Read the model definition and answer for the solid it produces. Units are mm, in the model's axes. Face numbers are marked on the shaded views. A direction names the side the tool comes from. Round coordinates to 2 decimals unless told otherwise and drop trailing zeros. Order: outer loops, then holes, each group sorted by start corner. A loop starts at its lowest first (then second) coordinate and runs counter-clockwise, first axis right, second up. Notation, with made-up numbers: M 25.5,-7 L 31.5,-7 A15 cw 31.5,14 Z; hole C 50.25,83.5 d5. An arc over 180 degrees is marked long. Answer as CSV lines item,"result".
```python
from build123d import *
from build123d.topology import SkipClean

# Parameters (mm, degrees)
SKETCH2_R           = 1.5
BOSS_EXTRUDE1_DEPTH = 3
SKETCH3_R           = 9.096048505
BOSS_EXTRUDE2_DEPTH = 1.2
FILLET1_R           = 1
CUT_EXTRUDE1_DEPTH  = 1.5
CUT_EXTRUDE2_START  = -1.5
CUT_EXTRUDE2_DEPTH  = 1.5
CUT_EXTRUDE3_DEPTH  = 5
MOVE_FACE1_BY       = 0.1
MOVE_FACE1_2_BY     = 0.1
MOVE_FACE1_3_BY     = 0.1


with BuildPart() as part:
    # Sketch2 → Boss-Extrude1 (new, symmetric)
    with BuildSketch(Plane(origin=(0, 0, 0), x_dir=(1, 0, 0), z_dir=(0, 1, 0))):
        with BuildLine():
            Line((-20.599560655, -3.593123858), (-21.028912901, -3.379903546))
            Line((-21.028912901, -3.379903546), (-21.254187526, 1.993220784))
            add(Edge.make_bspline(
                [(-21.254187526, 1.993220784), (-21.250081776, 2.377226096), (-21.195139063, 3.186038357), (-20.237966675, 3.678013728), (-19.626306607, 3.674971934), (-19.293061526, 3.554683236)],
                knots=[0.008573336, 0.008573336, 0.008573336, 0.008573336, 0.425411643, 0.645508579, 0.988655727, 0.988655727, 0.988655727, 0.988655727], degree=3))
            Line((-19.293061526, 3.554683236), (-19.293061526, -0.935875279))
            ThreePointArc((-19.293061526, -0.935875279), (-11.01478007, -15.867347151), (5.868677769, -18.402627716))
            ThreePointArc((5.868677769, -18.402627716), (8.914480471, -17.213611271), (11.689585214, -15.484603502))
            Line((11.689585214, -15.484603502), (16.248961374, -16.876941699))
            ThreePointArc((16.248961374, -16.876941699), (18.257558766, -15.774505508), (18.891422269, -13.572677609))
            Line((18.891422269, -13.572677609), (16.51986009, -9.867884272))
            ThreePointArc((16.51986009, -9.867884272), (18.681381592, -1.319406436), (16.449996012, 7.211101574))
            Line((16.449996012, 7.211101574), (17.928084104, 7.713187831))
            ThreePointArc((17.928084104, 7.713187831), (18.677006581, 8.400562387), (19.066466062, 9.339545863))
            Line((19.066466062, 9.339545863), (19.069212644, 11.701301235))
            ThreePointArc((19.069212644, 11.701301235), (18.53112158, 13.108816633), (17.413375201, 14.119402908))
            Line((17.413375201, 14.119402908), (16.248961374, 14.508827059))
            Line((16.248961374, 14.508827059), (17.314988377, 17.040275234))
            Line((17.314988377, 17.040275234), (-18.629227908, 17.040275234))
            Line((-18.629227908, 17.040275234), (-23.111573489, 16.669208858))
            ThreePointArc((-23.111573489, 16.669208858), (-24.534989581, 15.930034001), (-25.030823978, 14.404700893))
            Line((-25.030823978, 14.404700893), (-25.030823978, 12.70560175))
            ThreePointArc((-25.030823978, 12.70560175), (-24.756748057, 11.739888101), (-24.016241086, 11.062119787))
            Line((-24.016241086, 11.062119787), (-19.293061526, 9.00102042))
            Line((-19.293061526, 9.00102042), (-19.293061526, 5.839179653))
            Line((-19.293061526, 5.839179653), (-22.090684207, 5.839179653))
            ThreePointArc((-22.090684207, 5.839179653), (-22.935760928, 5.565442119), (-23.357392581, 4.783576625))
            Line((-23.357392581, 4.783576625), (-23.096619876, -3.253456456))
            Line((-23.096619876, -3.253456456), (-23.621531964, -3.576891157))
            ThreePointArc((-23.621531964, -3.576891157), (-23.831523214, -3.884927944), (-23.671952518, -4.221855504))
            Line((-23.671952518, -4.221855504), (-23.25143386, -4.644287186))
            Line((-23.25143386, -4.644287186), (-23.202937263, -6.523606801))
            add(Edge.make_bspline(
                [(-23.202937263, -6.523606801), (-23.190415125, -6.701394879), (-23.14585211, -7.158039831), (-22.604610265, -7.291644066), (-22.131088375, -7.301130698), (-21.611573501, -7.301182592), (-20.850084131, -7.060004854), (-20.915185829, -6.352757768), (-20.915665013, -6.081028816)],
                knots=[0, 0, 0, 0, 0.172348306, 0.293808545, 0.415161147, 0.571057182, 0.730620463, 1, 1, 1, 1], degree=3))
            Line((-20.915665013, -6.081028816), (-20.979073646, -4.568641575))
            Line((-20.979073646, -4.568641575), (-20.599560655, -4.155522335))
            ThreePointArc((-20.599560655, -4.155522335), (-20.467265038, -3.874323097), (-20.599560655, -3.593123858))
        make_face()
        with Locations(Location((16.153998691, -14.195749789, 0), (0, 0, 270))):
            Circle(SKETCH2_R, mode=Mode.SUBTRACT)
        with Locations(Location((-22.494848615, 13.810394624, 0), (0, 0, 270))):
            Circle(SKETCH2_R, mode=Mode.SUBTRACT)
        with Locations(Location((16.894563054, 10.777137226, 0), (0, 0, 270))):
            Circle(SKETCH2_R, mode=Mode.SUBTRACT)
    extrude(amount=BOSS_EXTRUDE1_DEPTH, both=True)

    # Sketch3 → Boss-Extrude2 (add)
    with BuildSketch(Plane(origin=(0, 3, 0), x_dir=(1, 0, 0), z_dir=(0, 1, 0))):
        with Locations(Location((3.73137128, -0.69899531, 0), (0, 0, 270))):
            Circle(SKETCH3_R)
    extrude(amount=BOSS_EXTRUDE2_DEPTH)

    # Fillet1
    fillet1_edges = [part.edges().sort_by_distance(p)[0] for p in [
        (3.73137128, 4.2, -8.397053195),
    ]]
    fillet(fillet1_edges, radius=FILLET1_R)

    # Sketch4 → Cut-Extrude1 (cut)
    with SkipClean():  # the faces are left unmerged after this step: merging them gives an invalid solid
        with BuildSketch(Plane(origin=(0, 3, 0), x_dir=(1, 0, 0), z_dir=(0, 1, 0))):
            Polygon((-19.293061526, 7.248655358), (-19.293061526, 22.083159944), (-29.904114882, 22.083159944), (-28.79317924, 8.663465276), align=None)
            with BuildLine():
                Line((17.65280475, 17.842473148), (14.40910217, 10.139793056))
                ThreePointArc((14.40910217, 10.139793056), (16.735981963, 6.675507155), (18.187015276, 2.762688645))
                Line((18.187015276, 2.762688645), (25.347732491, 2.045186791))
                Line((25.347732491, 2.045186791), (30.175625625, 15.043360613))
                Line((30.175625625, 15.043360613), (17.65280475, 17.842473148))
            make_face()
            with BuildLine():
                Line((17.279847396, -8.294754226), (24.575782686, -15.276129443))
                Line((24.575782686, -15.276129443), (17.279847396, -23.8721919))
                Line((17.279847396, -23.8721919), (10.670432719, -16.203678062))
                ThreePointArc((10.670432719, -16.203678062), (14.563628552, -12.741010549), (17.279847396, -8.294754226))
            make_face()
        extrude(amount=-CUT_EXTRUDE1_DEPTH, mode=Mode.SUBTRACT)

    # Sketch5 → Cut-Extrude2 (cut)
    with SkipClean():  # the faces are left unmerged after this step: merging them gives an invalid solid
        with BuildSketch(Plane.XZ.offset(3).offset(CUT_EXTRUDE2_START)):
            with BuildLine():
                Line((14.40910217, -10.139793056), (17.65280475, -17.842473148))
                Line((17.65280475, -17.842473148), (30.175625625, -15.043360613))
                Line((30.175625625, -15.043360613), (25.347732491, -2.045186791))
                Line((25.347732491, -2.045186791), (18.187015276, -2.762688645))
                ThreePointArc((18.187015276, -2.762688645), (16.735981963, -6.675507155), (14.40910217, -10.139793056))
            make_face()
            Polygon((-19.293061526, -22.083159944), (-19.293061526, -7.248655358), (-28.79317924, -8.663465276), (-29.904114882, -22.083159944), align=None)
            with BuildLine():
                Line((24.575782686, 15.276129443), (17.279847396, 23.8721919))
                Line((17.279847396, 23.8721919), (10.670432719, 16.203678062))
                ThreePointArc((10.670432719, 16.203678062), (14.563628552, 12.741010549), (17.279847396, 8.294754226))
                Line((17.279847396, 8.294754226), (24.575782686, 15.276129443))
            make_face()
        extrude(amount=CUT_EXTRUDE2_DEPTH, mode=Mode.SUBTRACT)

    # Sketch6 → Cut-Extrude3 (cut)
    with SkipClean():  # the faces are left unmerged after this step: merging them gives an invalid solid
        with BuildSketch(Plane(origin=(0, 3, 0), x_dir=(1, 0, 0), z_dir=(0, 1, 0))):
            Polygon((-19.293061526, -0.935875279), (-19.293061526, 7.436034842), (-28.419835781, 7.111305906), (-26.742069614, -11.668850866), (-19.293061526, -11.003377521), align=None)
        extrude(amount=-CUT_EXTRUDE3_DEPTH, mode=Mode.SUBTRACT)

    # Move Face1: a curved face moved inward by 0.1
    add(Solid.thicken(part.faces().sort_by_distance((16.153998691, 0, 12.695749789))[0], -MOVE_FACE1_BY), mode=Mode.SUBTRACT)

    # Move Face1 2: a curved face moved inward by 0.1
    add(Solid.thicken(part.faces().sort_by_distance((-22.494848615, 0, -15.310394624))[0], -MOVE_FACE1_2_BY), mode=Mode.SUBTRACT)

    # Move Face1 3: a curved face moved inward by 0.1
    add(Solid.thicken(part.faces().sort_by_distance((16.894563054, 0, -12.277137226))[0], -MOVE_FACE1_3_BY), mode=Mode.SUBTRACT)


solid = part.part
```
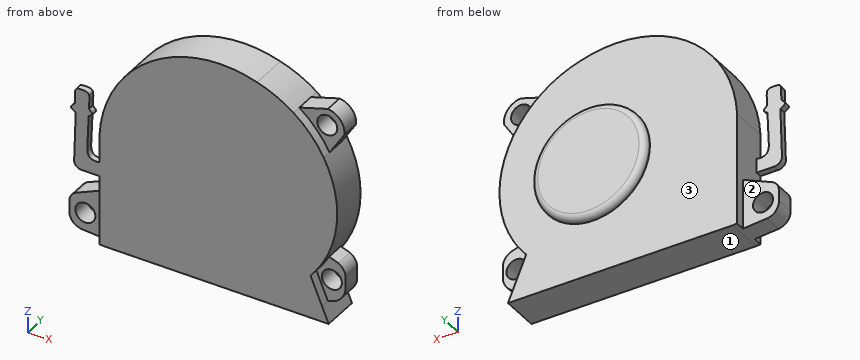
Item 1: A cutting plane is placed at A-A, the plane y = 2.25. Determine the outline of the cut face in (x, z), and give its area (3 significant figures).
Ans:
outline,"M -19.29,-16.99 L -18.63,-17.04 L 17.31,-17.04 L 14.41,-10.14 A17.7 ccw 5.87,18.4 A19.32 ccw -19.29,0.94 Z"
area,"1,200 mm2"
Item 2: A cutting plane is placed at B-B, the plane y = -0.75. Determine the outline of the cut face in (x, z), and give its area (3 significant figures).
Ans:
outline,"M -25.03,-14.4 A2.12 ccw -23.11,-16.67 L -18.63,-17.04 L 17.31,-17.04 L 16.25,-14.51 L 17.41,-14.12 A3.23 ccw 19.07,-11.7 L 19.07,-9.34 A2.36 ccw 17.93,-7.71 L 16.45,-7.21 A17.7 ccw 16.52,9.87 L 18.89,13.57 A2.98 ccw 16.25,16.88 L 11.69,15.48 A17.7 ccw 5.87,18.4 A19.32 ccw -19.29,0.94 L -19.29,-9 L -24.02,-11.06 A1.84 ccw -25.03,-12.71 Z; hole C -22.49,-13.81 d3.2; hole C 16.15,14.2 d3.2; hole C 16.89,-10.78 d3.2"
area,"1,260 mm2"
Item 3: A tool of negligible diameter and unlimited length cuts with its end or side. For the marked faces 1, 2 and 3, from which of +Z, -Z, +X, -X, +Y, -Y can it reach the whole face along a straight path? Write none if from no direction.
Ans:
face 1,"-Z, +X, -X, +Y, -Y"
face 2,"+Z, -Z, -X, +Y"
face 3,"+Y"
Item 4: Find the intervals of material crossed by probe 1 along Y at (x, z) = (7, -12); probe 2 along Z at (x, y) = (-0.5, -0.75); probe 3 along X at (y, z) = (-1.25, 14.5), in increasing order. Write a range as [from, to].
Ans:
probe 1,"[-3, 3]"
probe 2,"[-17.04, 19.31]"
probe 3,"[-12.76, 14.58], [17.72, 18.85]"
Item 5: Flat-ended cylindrical pins translate along their axes: pin 1 (0.5 mm diameter, centred on y = 0.5, z = -13.5, fed in from -X); pin 2 (3 mm diameter, centred on x = 16.15, z = 14.2, fed in from +Y); pin 3 (1.4 mm diameter, centred on x = -21, z = 2.5, fed in from +Y); pin 4 (6.5 mm diameter, centred on x = -21, z = -12, fed in from +Y). Find the tip coordinate at first contact, or state that the pin passes through.
Ans:
pin 1,"x = -25.03"
pin 2,"through"
pin 3,"y = -2"
pin 4,"y = 3"
